Autodesk Inventor part; units mm, degrees
ref_plane "YZ Plane" through (0, 0, 0) normal (1, 0, 0) x (0, 1, 0)
ref_plane "XZ Plane" through (0, 0, 0) normal (0, 1, 0) x (-1, 0, 0)
ref_plane "XY Plane" through (0, 0, 0) normal (0, 0, 1) x (1, 0, 0)
sketch "Sketch1" plane through (0, 0, 0) normal (0, 1, 0) x (-1, 0, 0)
  line L0 (0, 0) -> (50, 0)
  line L1 (50, 0) -> (50, -50)
  line L2 (50, -50) -> (0, -50)
  line L3 (0, -50) -> (0, 0)
  circle A0 centre (40.5, -9.5) radius 2
  circle A1 centre (25, -25) radius 11
  circle A2 centre (40.5, -40.5) radius 2
  circle A3 centre (9.5, -9.5) radius 2
  circle A4 centre (9.5, -40.5) radius 2
  dimension "d0" = 50
  dimension "d1" = 50
  dimension "d2" = 4
  dimension "d3" = 9.5
  dimension "d4" = 9.5
  dimension "d5" = 22
  dimension "d6" = 25
  dimension "d7" = 25
  dimension "d10" = 31
  dimension "d13" = 31
extrude "Extrusion1" add sketch "Sketch1" along normal blind 2
fillet "Fillet1" radius 10 4 edges at (0, 1, -50) (0, 1, 0) (-50, 1, -50) (-50, 1, 0)
sketch "Sketch2" plane through (0, 2, 0) normal (0, 1, 0) x (1, 0, 0)
  circle A0 centre (-40.5, 9.5) radius 2
  circle A1 centre (-40.5, 9.5) radius 6
  point P0 (0, 0)
  dimension "d19" = 12
extrude "Extrusion2" cut sketch "Sketch2" against normal blind 1
pattern_linear "Rectangular Pattern1" count 2 spacing 31 along (1, 0, 0) count 2 spacing 31 along (0, 0, -1) of "Extrusion2"
properties part number "NEMA17_FacePlate"
The model under review builds one solid part; all positions refer to its coordinate system, in mm. A direction names the side the tool comes from. Coordinates: 2 decimals unless noted, no trailing zeros. Loops run counter-clockwise (first coordinate to the right, second up) from the corner with the lowest first, then second, coordinate; pieces in that order, holes last. Notation, with made-up numbers: (10.25, 63.5) -> (56.25, 63.5) arc R20 ccw to (56.25, 82.5) -> close; hole circle Ø8 at (20.5, -29.75). An arc over 180 degrees is marked (long way). Answer as CSV lines item,"result".
Item 1: For L1, parallel to X at y = 1.2, z = -9.5; L2, parallel to Z at x = -40.5, y = 0.75, list the stretches that pass through material, from the lowest coordinate up.
Results below:
L1,"x = -49.99 to -46.5, -34.5 to -15.5, -3.5 to -0.01"
L2,"z = -49.99 to -42.5, -38.5 to -11.5, -7.5 to -0.01"
Item 2: Draft analysis for pull direction Z (two halves, no side actions). For faces 1 (the cylindrical face through (-9.066, 0.493, -38.548)), 2 (the cylindrical face through (-2.85, 1.01, -46.99)), 3 (the cylindrical face through (-3.01, 1.01, -2.85)), state which applies: +Z half, -Z half, draft (parallel to the pull), parting line (faces both ways), or undercut.
Results below:
face 1,"undercut"
face 2,"-Z half"
face 3,"+Z half"
Item 3: Take a section at B-B, the plane x = -25. State the section outline as (y, z) points.
Results below:
outline,"(0, -50) -> (2, -50) -> (2, -36) -> (0, -36) -> close; (0, -14) -> (2, -14) -> (2, 0) -> (0, 0) -> close"
Item 4: Insertion check: pin 1 (6 mm diameter, centred on x = -8.5, z = -42, fed in from +Y); pin 2 (1 mm diameter, centred on y = 0.5, z = -42.5, fed in from -X). Each pin has a flat end and moves straight along its axis. Give the tip position at first contact, or say it passes through.
Results below:
pin 1,"stops at y = 1"
pin 2,"stops at x = -49.8"
Item 5: Take a section at A-A, the plane y = 1.3. State the section outline as (x, z) points.
Results below:
outline,"(-50, -40) arc R10 ccw to (-40, -50) -> (-10, -50) arc R10 ccw to (0, -40) -> (0, -10) arc R10 ccw to (-10, 0) -> (-40, 0) arc R10 ccw to (-50, -10) -> close; hole circle Ø12 at (-40.5, -40.5); hole circle Ø12 at (-40.5, -9.5); hole circle Ø22 at (-25, -25); hole circle Ø12 at (-9.5, -40.5); hole circle Ø12 at (-9.5, -9.5)"
Item 6: Take a section at C-C, the plane z = -28.5. State the section outline as (x, y) points.
Results below:
outline,"(-50, 0) -> (-35.43, 0) -> (-35.43, 2) -> (-50, 2) -> close; (-14.57, 0) -> (0, 0) -> (0, 2) -> (-14.57, 2) -> close"
Item 7: Take a section at D-D, the plane z = -45.5. State the section outline as (x, y) points, and give its area (3 significant figures).
Results below:
outline,"(-48.35, 0) -> (-1.65, 0) -> (-1.65, 2) -> (-6.18, 2) -> (-6.18, 1) -> (-12.82, 1) -> (-12.82, 2) -> (-37.18, 2) -> (-37.18, 1) -> (-43.82, 1) -> (-43.82, 2) -> (-48.35, 2) -> close"
area,"80.1 mm2"
Item 8: Machinability: for faces 4 (the flat face through (0, 1, -25)), 5 (the flat face through (-10, 1, -38)), which of the approach directions +Z, -Z, +X, -X, +Y, -Y give a long, thin tool a straight path to every point of the face, cutting with its end or side? Answer none if there is none.
Results below:
face 4,"+Z, -Z, +X, +Y, -Y"
face 5,"+Y"
